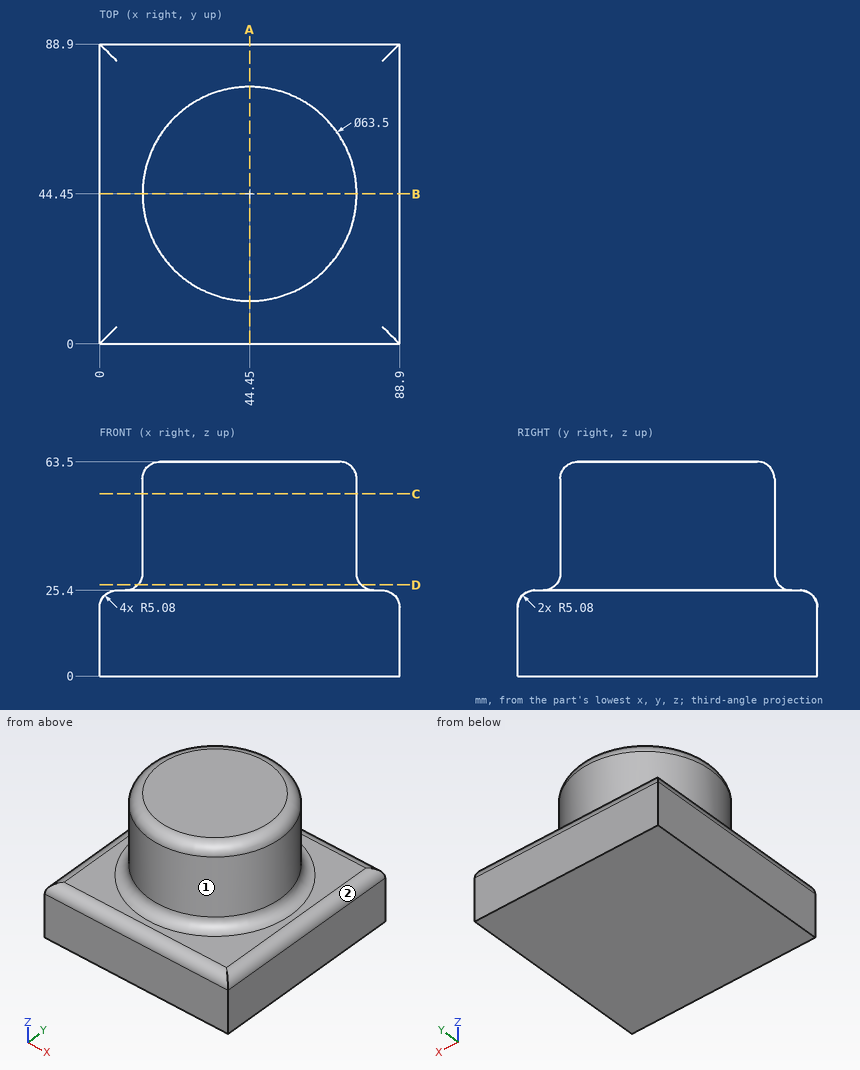
Can you work these out from the drawing? Everything is in mm from the part's minimum corner. A direction names the side the tool comes from. Give positions to 0.01 mm unless a question says otherwise; leave off trailing zeros. Write each loop counter-clockwise with the first axis right and the second up, starting at its lowest first coordinate (ties: lowest second). Pieces come first, ordered by that corner, then holes. Notation, with made-up numbers: (-26, 8) -> (-19, 8) arc R18 cw to (-19, 21) -> close; hole circle Ø2 at (-35, 39.5). An arc over 180 degrees is marked (long way). Write each question's results on one line, items separated by ' | '.
Item 1: On a 3-axis mill with a long thin cutter (end or side, diameter ignored), from which of +Z, -Z, +X, -X, +Y, -Y can I reach the whole of each face in a straight line? I mean the marked faces 1 and 2. Say none if no direction works.
Output:
face 1: +Z | face 2: +Z, +X, +Y, -Y
Item 2: If I drill on L1, parallel to Y at x = 12, z = 20.5; L2, parallel to Z at x = 84, y = 45; L3, parallel to Z at x = 77.5, y = 32.5, over which ranges is the centre line in solid material (lowest first)?
Output:
L1: y = 0 to 88.9 | L2: z = 0 to 25.4 | L3: z = 0 to 25.69
Item 3: Suppose I cut it at D-D on z = 27. Write out the boundary of the cut face in (x, y), plus the area to 3 significant figures.
Output:
outline: circle Ø66.26 at (44.45, 44.45) | area: 3,450 mm^2
Item 4: Suppose I cut it at C-C on z = 54. Write out the boundary of the cut face in (x, y).
Output:
outline: circle Ø63.5 at (44.45, 44.45)
Item 5: Suppose I cut it at A-A on x = 44.45. Write out the boundary of the cut face in (y, z).
Output:
outline: (0, 0) -> (88.9, 0) -> (88.9, 20.32) arc R5.08 ccw to (83.82, 25.4) -> (81.28, 25.4) arc R5.08 cw to (76.2, 30.48) -> (76.2, 58.42) arc R5.08 ccw to (71.12, 63.5) -> (17.78, 63.5) arc R5.08 ccw to (12.7, 58.42) -> (12.7, 30.48) arc R5.08 cw to (7.62, 25.4) -> (5.08, 25.4) arc R5.08 ccw to (0, 20.32) -> close
Item 6: For pin 1 Ø10 at (x, y) = (74, 28.5) entering from -Z; pin 2 Ø4 at (x, y) = (41, 76.5) entering from +Z; pin 3 Ø12 at (y, z) = (71.5, 28) entering from +X; pin 4 Ø5 at (x, y) = (21, 10.5) entering from +Z, each with a flat end and sliding along its axis, tell me the tip position at first contact or that it passes through.
Output:
pin 1: stops at z = 0 | pin 2: stops at z = 62.04 | pin 3: stops at x = 88.61 | pin 4: stops at z = 25.4
